from build123d import *

# Parameters (mm, degrees)
SKETCH_1_W           = 132
SKETCH_1_H           = 42
EXTRUDE_1_DEPTH      = 32
SKETCH_2_R           = 14.15
CUT_EXTRUDE_1_DEPTH  = 32
SKETCH_3_R           = 10.65
CUT_EXTRUDE_2_DEPTH  = 32
SKETCH_7_R           = 2.25
SKETCH_7_R_2         = 1.75
CUT_EXTRUDE_8_DEPTH  = 32
CUT_EXTRUDE_9_DEPTH  = 10
CUT_EXTRUDE_10_DEPTH = 6
SKETCH_10_R          = 1.25
CUT_EXTRUDE_26_DEPTH = 10


with BuildPart() as part:
    # 草图1 → 凸台-拉伸1 (new body)
    with BuildSketch(Plane.XY):
        with Locations((0, 1)):
            Rectangle(SKETCH_1_W, SKETCH_1_H)
    extrude(amount=EXTRUDE_1_DEPTH)

    # 草图2 → 切除-拉伸1 (cut)
    with BuildSketch(Plane(origin=(0, 0, 0), x_dir=(-1, 0, 0), z_dir=(0, 0, -1))):
        Circle(SKETCH_2_R)
    extrude(amount=-CUT_EXTRUDE_1_DEPTH, mode=Mode.SUBTRACT)

    # 草图3 → 切除-拉伸2 (cut)
    with BuildSketch(Plane(origin=(0, 0, 0), x_dir=(-1, 0, 0), z_dir=(0, 0, -1))):
        with Locations((-42, 0)):
            Circle(SKETCH_3_R)
        with Locations((42, 0)):
            Circle(SKETCH_3_R)
    extrude(amount=-CUT_EXTRUDE_2_DEPTH, mode=Mode.SUBTRACT)

    # 草图7 → 切除-拉伸8 (cut)
    with BuildSketch(Plane(origin=(0, 0, 0), x_dir=(-1, 0, 0), z_dir=(0, 0, -1))):
        with Locations((-13.435028843, 13.435028843)):
            Circle(SKETCH_7_R)
        with Locations((13.435028843, 13.435028843)):
            Circle(SKETCH_7_R)
        with Locations((13.435028843, -13.435028843)):
            Circle(SKETCH_7_R)
        with Locations((-13.435028843, -13.435028843)):
            Circle(SKETCH_7_R)
        with Locations((-18.998610576, 0)):
            Circle(SKETCH_7_R)
        with Locations((18.998532389, 0)):
            Circle(SKETCH_7_R)
        with Locations((30.686291501, 11.313708499)):
            Circle(SKETCH_7_R_2)
        with Locations((30.686291501, -11.313708499)):
            Circle(SKETCH_7_R_2)
        with Locations((53.313708499, 11.313708499)):
            Circle(SKETCH_7_R_2)
        with Locations((53.313708499, -11.313708499)):
            Circle(SKETCH_7_R_2)
        with Locations((-53.313708499, 11.313708499)):
            Circle(SKETCH_7_R_2)
        with Locations((-30.686291501, 11.313708499)):
            Circle(SKETCH_7_R_2)
        with Locations((-53.313708499, -11.313708499)):
            Circle(SKETCH_7_R_2)
        with Locations((-30.686291501, -11.313708499)):
            Circle(SKETCH_7_R_2)
    extrude(amount=-CUT_EXTRUDE_8_DEPTH, mode=Mode.SUBTRACT)

    # 草图8 → 切除-拉伸9 (cut)
    with BuildSketch(Plane(origin=(0, 0, 0), x_dir=(-1, 0, 0), z_dir=(0, 0, -1))):
        with BuildLine():
            Line((-13.417246364, 20.2), (13.417246364, 20.2))
            ThreePointArc((13.417246364, 20.2), (24.249341133, 0.178758535), (13.713588152, -20))
            Line((13.713588152, -20), (-13.713588152, -20))
            ThreePointArc((-13.713588152, -20), (-24.249341133, 0.178758535), (-13.417246364, 20.2))
        make_face()
    extrude(amount=-CUT_EXTRUDE_9_DEPTH, mode=Mode.SUBTRACT)

    # 草图9 → 切除-拉伸10 (cut)
    with BuildSketch(Plane(origin=(0, 0, 0), x_dir=(-1, 0, 0), z_dir=(0, 0, -1))):
        with BuildLine():
            Line((28.306936062, 16.25), (55.693063938, 16.25))
            ThreePointArc((55.693063938, 16.25), (57.0260191, 15.0260191), (58.25, 13.693063938))
            Line((58.25, 13.693063938), (58.25, -13.693063938))
            ThreePointArc((58.25, -13.693063938), (57.0260191, -15.0260191), (55.693063938, -16.25))
            Line((55.693063938, -16.25), (28.306936062, -16.25))
            ThreePointArc((28.306936062, -16.25), (26.9739809, -15.0260191), (25.75, -13.693063938))
            Line((25.75, -13.693063938), (25.75, 13.693063938))
            ThreePointArc((25.75, 13.693063938), (26.9739809, 15.0260191), (28.306936062, 16.25))
        make_face()
        with BuildLine():
            Line((-55.693063938, 16.25), (-28.306936062, 16.25))
            ThreePointArc((-28.306936062, 16.25), (-26.9739809, 15.0260191), (-25.75, 13.693063938))
            Line((-25.75, 13.693063938), (-25.75, -13.693063938))
            ThreePointArc((-25.75, -13.693063938), (-26.9739809, -15.0260191), (-28.306936062, -16.25))
            Line((-28.306936062, -16.25), (-55.693063938, -16.25))
            ThreePointArc((-55.693063938, -16.25), (-57.0260191, -15.0260191), (-58.25, -13.693063938))
            Line((-58.25, -13.693063938), (-58.25, 13.693063938))
            ThreePointArc((-58.25, 13.693063938), (-57.0260191, 15.0260191), (-55.693063938, 16.25))
        make_face()
    extrude(amount=-CUT_EXTRUDE_10_DEPTH, mode=Mode.SUBTRACT)

    # 草图10 → 切除-拉伸26 (cut)
    with BuildSketch(Plane(origin=(0, 22, 0), x_dir=(1, 0, 0), z_dir=(0, 1, 0))):
        with Locations((25, -25)):
            Circle(SKETCH_10_R)
        with Locations((61, -25)):
            Circle(SKETCH_10_R)
        with Locations((-25, -25)):
            Circle(SKETCH_10_R)
        with Locations((-61, -25)):
            Circle(SKETCH_10_R)
        with Locations((61, -7)):
            Circle(SKETCH_10_R)
        with Locations((-61, -7)):
            Circle(SKETCH_10_R)
    extrude(amount=-CUT_EXTRUDE_26_DEPTH, mode=Mode.SUBTRACT)


solid = part.part
Source: CAD feature listing. Evaluate the final solid. Frame: model axes, mm. A direction names the side the tool comes from. Round coordinates to 2 decimals unless told otherwise and drop trailing zeros. Loops run counter-clockwise (first coordinate to the right, second up) from the corner with the lowest first, then second, coordinate; pieces in that order, holes last.
Q1. Access query for faces 4 (the face through (0, 20.2, 5)), 5 (the face through (26.99, 15.04, 2.96)), 6 (the face through (-25, 12, 25)). Directions: +Z, -Z, +X, -X, +Y, -Y. A direction counts if a zero-diameter tool reaches every point of the face in a straight line with its end or side. Return the directions, or none.
Q2. Section B-B, the plane z = 2. Return loops of the section in (x, y), plus the area to 3 significant figures.
Q3. Section C-C, the plane x = 47. Return loops of the section in (y, z), plus the area to 3 significant figures.
Q4. First-contact query: P1, Ø16, axis at x = 48.5, y = -5, coming from the -Z side; P2, Ø1.5, axis at x = -61, z = 25, coming from the +Y side. Flat tips, straight axial feed; report the tip coordinate or a pass-through.
Q5. Ray query, line 1 (Z direction, x = -61, y = 17); line 2 (Y direction, x = 41.5, z = 26.5); line 3 (X direction, y = -7.5, z = 2). Return the intervals inside material, ascending.
Q6. Section A-A, the plane x = -61. Return loops of the section in (y, z).
Q7. Section D-D, the plane z = 19.5. State how many separate pieces and enclosed holes the cut face has, plus the area to 3 significant figures.
Q8. Mould query, pull axis X, two halves, no side actions, for faces 1 (the face through (42, 16.25, 3)), 2 (the face through (-66, 1, 16)), 3 (the face through (5, 21, 0)). Classes: pulls with the +X half, pulls with the -X half, needs draft (parallel to the pull), parting line crosses it, or undercut.
Solutions:
1. face 4: -Z, -Y
1. face 5: -Z
1. face 6: +Y
2. outline: (-66, -20) - (-13.71, -20) arc R24.25 cw to (-13.42, 20.2) - (13.42, 20.2) arc R24.25 cw to (13.71, -20) - (66, -20) - (66, 22) - (-66, 22) - close; hole (-58.25, -13.69) arc R21.25 ccw to (-55.69, -16.25) - (-28.31, -16.25) arc R21.25 ccw to (-25.75, -13.69) - (-25.75, 13.69) arc R21.25 ccw to (-28.31, 16.25) - (-55.69, 16.25) arc R21.25 ccw to (-58.25, 13.69) - close; hole (25.75, -13.69) arc R21.25 ccw to (28.31, -16.25) - (55.69, -16.25) arc R21.25 ccw to (58.25, -13.69) - (58.25, 13.69) arc R21.25 ccw to (55.69, 16.25) - (28.31, 16.25) arc R21.25 ccw to (25.75, 13.69) - close
2. area: 1,760 mm2
3. outline: (-20, 0) - (-16.25, 0) - (-16.25, 6) - (-9.4, 6) - (-9.4, 32) - (-20, 32) - close; (9.4, 6) - (16.25, 6) - (16.25, 0) - (22, 0) - (22, 32) - (9.4, 32) - close
3. area: 660 mm2
4. P1: stops at z = 6
4. P2: stops at y = 12
5. line 1: z = 0 to 5.75, 8.25 to 23.75, 26.25 to 32
5. line 2: y = -20 to -10.64, 10.64 to 22
5. line 3: x = -66 to -58.25, -25.75 to -23.06, 23.06 to 25.75, 58.25 to 66
6. outline: (-20, 0) - (22, 0) - (22, 5.75) - (12, 5.75) - (12, 8.25) - (22, 8.25) - (22, 23.75) - (12, 23.75) - (12, 26.25) - (22, 26.25) - (22, 32) - (-20, 32) - close
7. separate pieces: 1
7. enclosed holes: 17
7. area: 4,030 mm2
8. face 1: undercut
8. face 2: pulls with the -X half
8. face 3: needs draft
